from build123d import *

# Parameters (mm, degrees)
F0_R     = 4.25
F1_DEPTH = 19
F2_R     = 9.5
F2_R_2   = 4.25
F3_DEPTH = 5
F4_R     = 6
F5_DEPTH = 50
F7_DEPTH = 15


with BuildPart() as f1:
    # F0 (on Front) → F1 (new body)
    with BuildSketch(Plane.XZ):
        Circle(F0_R)
    extrude(amount=F1_DEPTH)

    # F2 (on face) → F3 (join)
    with BuildSketch(Plane.XZ.offset(19)):
        Circle(F2_R)
        Circle(F2_R_2, mode=Mode.SUBTRACT)
        Circle(F2_R_2)
    extrude(amount=F3_DEPTH)

    # F4 (on face) → F5 (join)
    with BuildSketch(Plane.XZ.offset(24)):
        Circle(F4_R)
    extrude(amount=F5_DEPTH)

    # F6 (on face) → F7 (join)
    with BuildSketch(Plane.XZ.offset(74)):
        Polygon((6, -3.4641016151), (6, 3.4641016151), (0, 6.9282032303), (-6, 3.4641016151), (-6, -3.4641016151), (0, -6.9282032303), align=None)
    extrude(amount=F7_DEPTH)


solid = f1.part
Input: part model. Units: mm. Frame: model coordinates. A direction names the side the tool comes from. Round coordinates to 2 decimals unless told otherwise and drop trailing zeros. Loops run counter-clockwise (first coordinate to the right, second up) from the corner with the lowest first, then second, coordinate; pieces in that order, holes last. Notation, with made-up numbers: (-31.5, 6.25) -> (-24.5, 6.25) arc R22 ccw to (-24.5, 29.25) -> close; hole circle Ø11 at (-34.75, 36). An arc over 180 degrees is marked (long way). Answer as a JSON object with one key per item and string values. Group by question number.
1) Draft query along Y for faces 5 (the flat face through (5.4, -74, 3)), 6 (the flat face through (0, -74, 6.2)), 7 (the flat face through (0, 0, 0)), 8 (the flat face through (-2.96, -81.4, 5.22)). Return one class per face: +Y half, -Y half, draft (parallel to the pull), parting line (faces both ways), or undercut.
2) Pin query (flat end, axial travel): pin 1 (1.5 mm diameter, centred on x = 4, z = -7, fed in from -Y); pin 2 (8 mm diameter, centred on x = 1.5, y = -33.5, fed in from -Z); pin 3 (1 mm diameter, centred on x = -2, y = -20, fed in from -Z); pin 4 (10 mm diameter, centred on x = 0.5, z = 2.5, fed in from +Y). Return the tip coordinate at first contact, or that it passes through.
3) Section query A-A on y = -10. Output: boundary loops of the cut face in (x, z).
4) Reachability of faces 1 (the flat face through (0, -74, -6.2)), 2 (the flat face through (-3.042, -81.395, -5.172)), 3 (the flat face through (-5.4, -74, 3)), 4 (the flat face through (4, -19, -2)) from +Z, -Z, +X, -X, +Y, -Y: full face, straight path, thin tool, end or side. Return the list, or none.
5) Section query B-B on x = -1.75. Output: boundary loops of the cut face in (y, z).
6) Section query D-D on y = -32. Output: boundary loops of the cut face in (x, z), plus the area to 3 significant figures.
7) Ray query, L1, parallel to Z at x = -4.25, y = -66; L2, parallel to Z at x = 3, y = -77; L3, parallel to Y at x = 4.25, z = 5.5. Return the intervals inside material, ascending.
8) Section query C-C on y = -75. Output: boundary loops of the cut face in (x, z), plus the area to 3 significant figures.
Reply:
{
 "1": {"face 5": "undercut", "face 6": "undercut", "face 7": "+Y half", "face 8": "draft"},
 "2": {"pin 1": "stops at y = -24", "pin 2": "stops at z = -6", "pin 3": "stops at z = -9.38", "pin 4": "stops at y = 0"},
 "3": {"outline": "circle Ø8.5 at (0, 0)"},
 "4": {"face 1": "-Z", "face 2": "-Z, -X, -Y", "face 3": "+Z, -X", "face 4": "+Y"},
 "5": {"outline": "(-89, -5.92) -> (-74, -5.92) -> (-74, -5.74) -> (-24, -5.74) -> (-24, -9.34) -> (-19, -9.34) -> (-19, -3.87) -> (0, -3.87) -> (0, 3.87) -> (-19, 3.87) -> (-19, 9.34) -> (-24, 9.34) -> (-24, 5.74) -> (-74, 5.74) -> (-74, 5.92) -> (-89, 5.92) -> close"},
 "6": {"outline": "circle Ø12 at (0, 0)", "area": "113 mm2"},
 "7": {"L1": "z = -4.24 to 4.24", "L2": "z = -5.2 to 5.2", "L3": "y = -24 to -19"},
 "8": {"outline": "(-6, -3.46) -> (0, -6.93) -> (6, -3.46) -> (6, 3.46) -> (0, 6.93) -> (-6, 3.46) -> close", "area": "125 mm2"}
}
